```python
from build123d import *

# Parameters (mm, degrees)
F0_W          = 26.7619055467
F0_H          = 8
F0_W_2        = 2.3985728621
F0_H_2        = 18.6882130802
F1_DEPTH      = 3
F3_DEPTH      = 5
F3_DEPTH_BACK = 7
F5_DEPTH      = 3


with BuildPart() as f1:
    # F0 (on Top) → F1 (new body)
    with BuildSketch(Plane.XY):
        Rectangle(F0_W, F0_H)
        with BuildLine():
            Line((52.8560965785, 21.0423569454), (13.3809527733, 4))
            Line((13.3809527733, 4), (13.3809527733, -4))
            Line((13.3809527733, -4), (52.8560965785, -21.0423569454))
            ThreePointArc((52.8560965785, -21.0423569454), (57.5848119408, -20.6297501175), (59.837911278, -16.4518874164))
            add(Edge.make_bspline(
                [(59.837911278, 16.4518874164), (61.2770561129, 11.6345916109), (64.1553457826, 0), (61.2770561129, -11.6345916109), (59.837911278, -16.4518874164)],
                knots=[0, 0, 0, 0, 0.5, 1, 1, 1, 1], degree=3))
            ThreePointArc((59.837911278, 16.4518874164), (57.5848119408, 20.6297501175), (52.8560965785, 21.0423569454))
        make_face()
        with Locations((55.1606826484, 0)):
            Rectangle(F0_W_2, F0_H_2, mode=Mode.SUBTRACT)
    extrude(amount=F1_DEPTH)

    # F2 (on face) → F3 (join, two sides)
    with BuildSketch(Plane.XY.offset(3)) as f3_sk:
        with BuildLine():
            ThreePointArc((65.3452423009, -29.7888193663), (68.8807762069, -28.3243532722), (70.3452423009, -24.7888193663))
            Line((70.3452423009, -24.7888193663), (70.3452423009, 16.4658156037))
            ThreePointArc((70.3452423009, 16.4658156037), (68.8807762069, 20.0013495097), (65.3452423009, 21.4658156037))
            Line((65.3452423009, 21.4658156037), (18.3809527733, 21.4658156037))
            ThreePointArc((18.3809527733, 21.4658156037), (14.8454188674, 20.0013495097), (13.3809527733, 16.4658156037))
            Line((13.3809527733, 16.4658156037), (13.3809527733, -19.452085589))
            add(Edge.make_bspline(
                [(13.3809527733, -19.452085589), (13.3809527733, -21.0615276884), (16.7556266537, -26.514923688), (23.4789476527, -29.7888193663), (40.723754061, -29.7888193663)],
                knots=[0, 0, 0, 0, 0.3158208681, 1, 1, 1, 1], degree=3))
            Line((40.723754061, -29.7888193663), (40.723754061, -21.0617277771))
            Line((40.723754061, -21.0617277771), (61.6181507117, -21.0617277771))
            Line((61.6181507117, -21.0617277771), (61.6181507117, -29.7888193663))
            Line((61.6181507117, -29.7888193663), (65.3452423009, -29.7888193663))
        make_face()
    extrude(amount=F3_DEPTH)
    extrude(f3_sk.sketch, amount=-F3_DEPTH_BACK)

    # F4 (on face) → F5 (join, through all)
    with BuildSketch(Plane.XY.offset(3)):
        Polygon((-13.3809527733, -4), (-13.3809527733, 4), (-23.397071287, 0), (-22.625775183, -1.9313482969), align=None)
    extrude(amount=-F5_DEPTH)


solid = f1.part
```
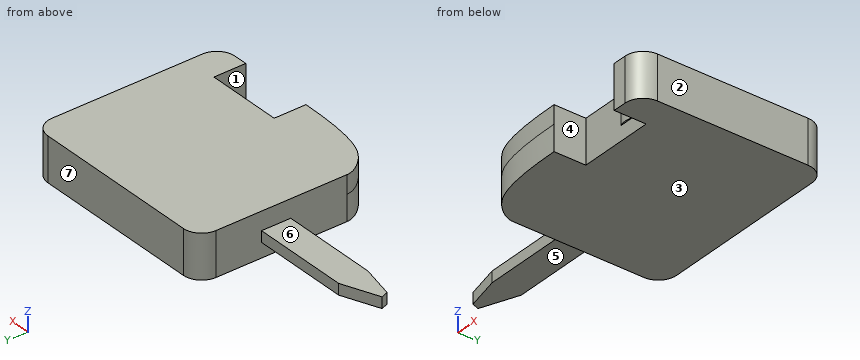
Model file for the job. Use its own axes, mm. Face numbers are marked on the shaded views. A direction names the side the tool comes from. Coordinates: 2 decimals unless noted, no trailing zeros. Write each loop counter-clockwise with the first axis right and the second up, starting at its lowest first coordinate (ties: lowest second). Pieces come first, ordered by that corner, then holes. Notation, with made-up numbers: (85.5, 4.25) - (105.5, 4.25) arc R17 cw to (105.5, 12.25) - close; hole circle Ø2 at (33.25, 87.5). An arc over 180 degrees is marked (long way). One line per item, written item: value. Start each with the question number.
1. Probe line 1 (X direction, y = 15, z = 2.25); line 2 (Y direction, x = 42, z = 7.25); line 3 (Z direction, x = 8, y = -2). List the from-to ranges inside material, lowest first. Write a range as from..to.
2. Flat gauge pins, fed straight in: pin 1 (2 mm diameter, centred on x = 36, z = 2, fed in from -Y); pin 2 (3.5 mm diameter, centred on x = -2.5, z = 1, fed in from +Y); pin 3 (3.5 mm diameter, centred on x = 1.5, z = 1.5, fed in from -Y). Where does each tip first touch, or does it go through?
3. Mould opens along X. For the marked faces 1, 2 and 3 say: released by +X, released by -X, zero draft, split by the parting line, or undercut.
4. Slice it at B-B (x = -4). Write the cut outline in (y, z), plus the area to 3 significant figures.
5. Slice it at C-C (y = 1). Write the cut outline in (x, z).
6. Tool access for the marked faces 4, 5, 6 and 7: list every direction of +Z, -Z, +X, -X, +Y, -Y with a clear straight run to the whole face (end or side of a thin tool).
7. Slice it at A-A (y = -16.5). Write the cut outline in (x, z), plus the area to 3 significant figures.
Answers below:
1. line 1: x = 13.38..70.35
1. line 2: y = -21.06..21.47
1. line 3: z = 0..3
2. pin 1: stops at y = -29.75
2. pin 2: stops at y = 4
2. pin 3: stops at y = -4
3. face 1: undercut
3. face 2: released by +X
3. face 3: zero draft
4. outline: (-4, 0) - (4, 0) - (4, 3) - (-4, 3) - close
4. area: 24.0 mm^2
5. outline: (-20.89, 0) - (13.38, 0) - (13.38, -4) - (70.35, -4) - (70.35, 8) - (13.38, 8) - (13.38, 3) - (-20.89, 3) - close
6. face 4: +Z, -Z, -Y
6. face 5: -Z, -X, +Y, -Y
6. face 6: +Z, -X, +Y, -Y
6. face 7: +Z, -Z, +X, -X, +Y
7. outline: (13.38, -4) - (70.35, -4) - (70.35, 8) - (13.38, 8) - close
7. area: 684 mm^2
